Here's the drawing with two shaded views (mm, measured from the low corner). I have some questions. A direction names the side the tool comes from. Round coordinates to 2 decimals unless told otherwise and drop trailing zeros. Order: outer loops, then holes, each group sorted by start corner. A loop starts at its lowest first (then second) coordinate and runs counter-clockwise, first axis right, second up. Notation, with made-up numbers: (-21, 79) -> (-5, 79) arc R12 cw to (-5, 95) -> close; hole circle Ø5 at (63, 62). An arc over 180 degrees is marked (long way). One line per question, with ' | ' between items.
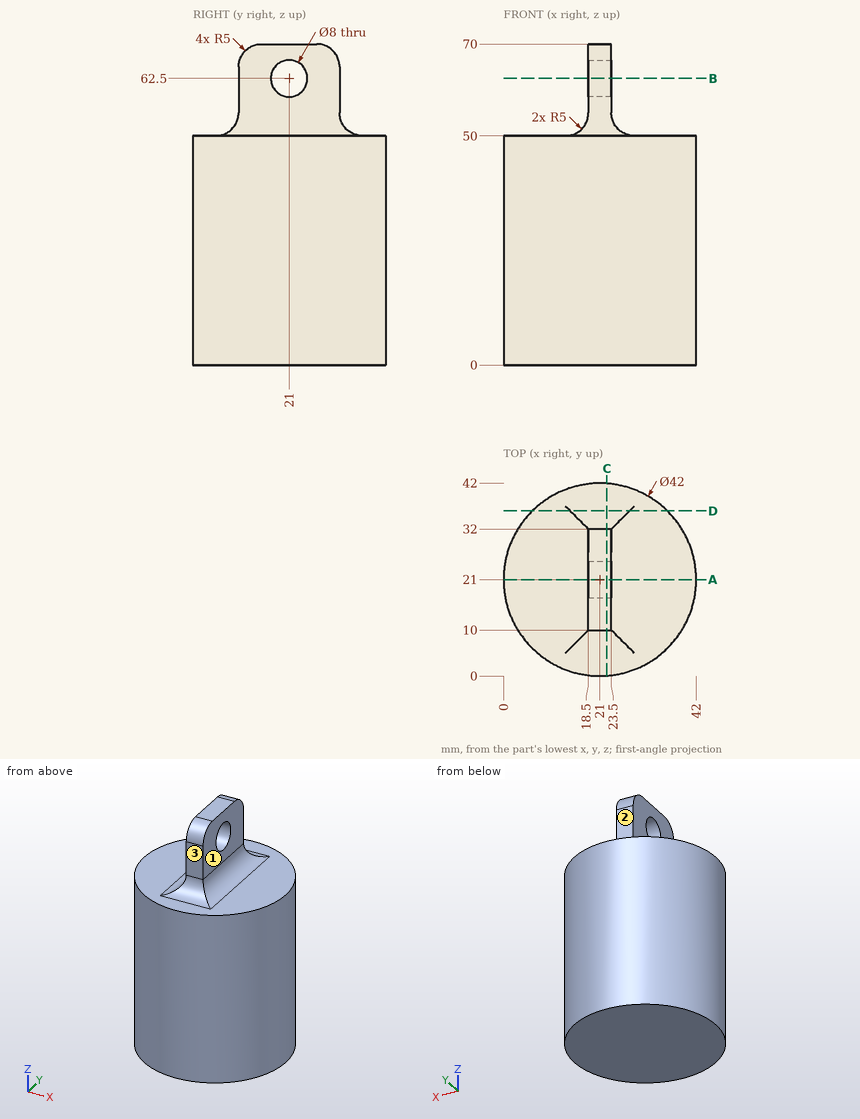
1. On a 3-axis mill with a long thin cutter (end or side, diameter ignored), from which of +Z, -Z, +X, -X, +Y, -Y can I reach the whole of each face in a straight line? I mean the marked faces 1, 2 and 3. Say none if no direction works.
From the geometry:
face 1: +Z, +X, +Y, -Y | face 2: +Z, +X, -X, +Y | face 3: +Z, +X, -X, -Y
2. I want a section at B-B on z = 62.5. List the corners of the cut face in (x, y) for me.
From the geometry:
outline: (18.5, 10) -> (23.5, 10) -> (23.5, 17) -> (18.5, 17) -> close; (18.5, 25) -> (23.5, 25) -> (23.5, 32) -> (18.5, 32) -> close
3. I need wall thicknesses on probe 1 along Y at (x, z) = (20.6, 62.5); probe 2 along Z at (x, y) = (34.5, 17.5); probe 3 along Y at (x, z) = (21.5, 58). Which ranges of each line are inside material? Lowest first, please.
From the geometry:
probe 1: y = 10 to 17, 25 to 32 | probe 2: z = 0 to 50 | probe 3: y = 10 to 32
4. I want a section at A-A on y = 21. List the corners of the cut face in (x, z) for me.
From the geometry:
outline: (0, 0) -> (42, 0) -> (42, 50) -> (28.5, 50) arc R5 cw to (23.5, 55) -> (23.5, 58.5) -> (18.5, 58.5) -> (18.5, 55) arc R5 cw to (13.5, 50) -> (0, 50) -> close; (18.5, 66.5) -> (23.5, 66.5) -> (23.5, 70) -> (18.5, 70) -> close
5. I want a section at C-C on x = 22.5. List the corners of the cut face in (y, z) for me.
From the geometry:
outline: (0.05, 0) -> (41.95, 0) -> (41.95, 50) -> (37, 50) arc R5 cw to (32, 55) -> (32, 65) arc R5 ccw to (27, 70) -> (15, 70) arc R5 ccw to (10, 65) -> (10, 55) arc R5 cw to (5, 50) -> (0.05, 50) -> close; hole circle Ø8 at (21, 62.5)
6. I want a section at D-D on y = 36. List the corners of the cut face in (x, z) for me.
From the geometry:
outline: (6.3, 0) -> (35.7, 0) -> (35.7, 50) -> (28.5, 50) arc R5 cw to (27.5, 50.1) -> (14.5, 50.1) arc R5 cw to (13.5, 50) -> (6.3, 50) -> close
7. I'm going to push flat-ended pins straight in: pin 1 (4.5 mm diameter, centred on y = 24, z = 65.5, fed in from +X); pin 2 (2 mm diameter, centred on y = 18, z = 46, fed in from +X); pin 3 (1.5 mm diameter, centred on x = 22, z = 58, fed in from +Y). Where does each tip first touch, or does it pass through?
From the geometry:
pin 1: stops at x = 23.5 | pin 2: stops at x = 41.9 | pin 3: stops at y = 32
